```python
from build123d import *

# Parameters (mm, degrees)
BOSS_EXTRUDE1_DEPTH = 1.5875
SKETCH2_R           = 6.35
CUT_EXTRUDE1_DEPTH  = 200.716179568
FILLET1_R           = 12.7


with BuildPart() as part:
    # Sketch1 → Boss-Extrude1 (new body)
    with BuildSketch(Plane.XY):
        with BuildLine():
            Line((-124.506849283, -39.770231507), (-119.474980228, -87.671358692))
            add(Edge.make_bspline(
                [(-56.3280252, -154.902468877), (-56.346476044, -154.899600353), (-56.402884517, -154.890830617), (-56.611080033, -154.858170111), (-57.104136424, -154.77889222), (-58.050896577, -154.617474356), (-60.354414853, -154.185740423), (-63.388938266, -153.485638357), (-67.010951192, -152.444549796), (-70.219086063, -151.362943176), (-73.446369967, -150.103845866), (-76.612996137, -148.694555998), (-79.712216879, -147.138105291), (-82.737433419, -145.437839357), (-85.682209143, -143.597409415), (-88.540283438, -141.620764011), (-91.305584556, -139.512139868), (-93.972242223, -137.276052336), (-96.534599628, -134.917285272), (-98.987224972, -132.440880464), (-101.324922461, -129.852126585), (-103.542742806, -127.156547725), (-105.635993175, -124.359891507), (-107.600246622, -121.468116813), (-109.431350973, -118.487381131), (-111.125437151, -115.424027557), (-112.678926942, -112.284571448), (-114.088540191, -109.075686767), (-115.351301396, -105.804192123), (-116.464545718, -102.477036535), (-117.425924357, -99.101284939), (-118.233409317, -95.684103469), (-118.885297518, -92.232744524), (-119.242744402, -89.7206526), (-119.408317309, -88.286030012), (-119.442476963, -87.975658316), (-119.45920335, -87.820433155), (-119.468609128, -87.731931499), (-119.473836089, -87.682236519), (-119.474980228, -87.671358692)],
                knots=[0, 0, 0, 0, 0.000570634, 0.001744558, 0.006440232, 0.015831442, 0.031091736, 0.078042667, 0.110904268, 0.146108785, 0.181308268, 0.216502219, 0.251690199, 0.286871835, 0.322046819, 0.357214911, 0.392375937, 0.427529794, 0.462676442, 0.497815906, 0.532948271, 0.568073682, 0.603192339, 0.638304491, 0.673410436, 0.708510515, 0.743605108, 0.77869463, 0.813779526, 0.84886027, 0.88393736, 0.919011312, 0.954082662, 0.989151956, 0.994996677, 0.997334555, 0.998503491, 0.999672426, 1, 1, 1, 1], degree=3))
            Line((-56.3280252, -154.902468877), (-48.306849283, -156.147611733))
            Line((-48.306849283, -156.147611733), (-48.306849283, -39.770231507))
            Line((-48.306849283, -39.770231507), (-124.506849283, -39.770231507))
        make_face()
    extrude(amount=BOSS_EXTRUDE1_DEPTH)

    # Sketch2 → Cut-Extrude1 (cut, through all)
    with BuildSketch(Plane(origin=(0, 0, 0), x_dir=(-1, 0, 0), z_dir=(0, 0, -1))):
        with Locations((67.356849283, -103.270231507)):
            Circle(SKETCH2_R)
        with Locations((92.756849283, -103.270231507)):
            Circle(SKETCH2_R)
        with BuildLine():
            ThreePointArc((87.994349283, -68.345231507), (87.954154998, -67.547441621), (87.833979216, -66.757731507))
            Line((87.833979216, -66.757731507), (86.406849283, -66.757731507))
            Line((86.406849283, -66.757731507), (86.406849283, -69.932731507))
            Line((86.406849283, -69.932731507), (87.833979216, -69.932731507))
            ThreePointArc((87.833979216, -69.932731507), (87.954154998, -69.143021393), (87.994349283, -68.345231507))
        make_face()
        with BuildLine():
            Line((86.406849283, -66.757731507), (87.833979216, -66.757731507))
            ThreePointArc((87.833979216, -66.757731507), (72.119349283, -68.345231507), (87.833979216, -69.932731507))
            Line((87.833979216, -69.932731507), (86.406849283, -69.932731507))
            Line((86.406849283, -69.932731507), (86.406849283, -66.757731507))
        make_face()
        with BuildLine():
            Line((89.581849283, -69.932731507), (89.581849283, -66.757731507))
            Line((89.581849283, -66.757731507), (87.833979216, -66.757731507))
            ThreePointArc((87.833979216, -66.757731507), (87.954154998, -67.547441621), (87.994349283, -68.345231507))
            ThreePointArc((87.994349283, -68.345231507), (87.954154998, -69.143021393), (87.833979216, -69.932731507))
            Line((87.833979216, -69.932731507), (89.581849283, -69.932731507))
        make_face()
    extrude(amount=-CUT_EXTRUDE1_DEPTH, mode=Mode.SUBTRACT)

    # Fillet1
    fillet1_edges = [part.edges().sort_by_distance(p)[0] for p in [
        (-48.306849283, -39.770231507, 0.79375),
        (-48.306849283, -156.147611733, 0.79375),
    ]]
    fillet(fillet1_edges, radius=FILLET1_R)


solid = part.part
```
Could you check a few things on this model? Use its own coordinates, in mm. Coordinates: 2 decimals unless noted, no trailing zeros. Write each loop counter-clockwise with the first axis right and the second up, starting at its lowest first coordinate (ties: lowest second). Pieces come first, ordered by that corner, then holes. Notation, with made-up numbers: (-6, 17) -> (18, 17) arc R16 ccw to (18, 41) -> close; hole circle Ø2 at (-33, -5.5). An arc over 180 degrees is marked (long way). One line per question, with ' | ' between items. Start each with the question number.
1. Thinking about a two-plate mould opening in X: for faces 1 (the face through (-52.13, -43.39, 0.8)), 2 (the face through (-65.98, -109.47, 0.78)), 3 (the face through (-78, -96, 1.588)), 4 (the face through (-95.69, -108.9, 0.78)), which applies, pulls with the +X half, pulls with the -X half, needs draft (parallel to the pull), parting line crosses it, or undercut?
2. If we section it at B-B (z = 1): Count the separate pieces of the cut face and the enclosed holes in it, and give its area (3 significant figures).
3. Please list where these lines run through material, in increasing order: line 1 along X through (y, z) = (-101.5, 0.8); line 2 along Y through (x, z) = (-89, 0.6); line 3 along X through (y, z) = (-106, 0.25).
4. If we section it at A-A (y = -71.5): Please give me the cut outline in (x, z).
Return value:
1) face 1: pulls with the +X half | face 2: undercut | face 3: needs draft | face 4: undercut
2) separate pieces: 1 | enclosed holes: 3 | area: 6,640 mm²
3) line 1: x = -116.73 to -98.86, -86.66 to -73.46, -61.26 to -48.31 | line 2: y = -141.25 to -108.39, -98.15 to -69.93, -66.76 to -39.77 | line 3: x = -115.25 to -98.49, -87.02 to -73.09, -61.62 to -48.31
4) outline: (-121.17, 0) -> (-87.34, 0) -> (-87.34, 1.59) -> (-121.17, 1.59) -> close; (-72.77, 0) -> (-48.31, 0) -> (-48.31, 1.59) -> (-72.77, 1.59) -> close
